Build history of the part. All positions in model axes, mm. Round coordinates to 2 decimals unless told otherwise and drop trailing zeros. Loops run counter-clockwise (first coordinate to the right, second up) from the corner with the lowest first, then second, coordinate; pieces in that order, holes last. Notation, with made-up numbers: (-10.75, 85.25) - (21.25, 85.25) arc R10 cw to (21.25, 97.25) - close; hole circle Ø7 at (5.5, 41.5). An arc over 180 degrees is marked (long way). Put each result on its own line as item: value. Start each with the question number.
Autodesk Fusion 360 part; units mm, degrees
sketch "Esquisse3" plane through (0, 0, 0) normal (0, 1, 0) x (1, 0, 0)
  line L0 (-32.5, 271.1708) -> (-7.5, 296.1708)
  line L1 (-32.5, 261.1708) -> (127.5, 261.1708) construction
  line L2 (127.5, 216.1708) -> (-32.5, 216.1708) construction
  circle A0 centre (20, 261.1708) radius 3
  line L3 (-7.5, 296.1708) -> (102.5, 296.1708)
  circle A1 centre (89.5, 194.6708) radius 3
  line L4 (-32.5, 236.1708) -> (127.5, 236.1708) construction
  line L5 (0, -4.6657) -> (95, -4.6657)
  circle A2 centre (89.5, 236.1708) radius 3
  line L6 (47.5, 23.552) -> (47.5, 296.1708)
  circle A3 centre (5.5, 194.6708) radius 3
  line L7 (47.5, 30.3343) -> (47.5, -4.6657) construction
  line L8 (-44.913, 194.6708) -> (139.913, 194.6708) construction
  line L9 (-80, 133.8984) -> (0, -4.6657)
  line L10 (95, -4.6657) -> (175, 133.8984)
  line L11 (23.75, 67.2637) -> (23.75, -4.6657) construction
  line L12 (71.25, 67.8004) -> (71.25, 0) construction
  line L13 (-32.5, 216.1708) -> (-80, 133.8984)
  line L14 (127.5, 271.1708) -> (127.5, 216.1708)
  line L15 (102.5, 296.1708) -> (127.5, 271.1708)
  line L16 (-32.5, 216.1708) -> (-32.5, 271.1708)
  line L17 (-32.5, 271.1708) -> (127.5, 271.1708) construction
  line L18 (-20.2073, 30.3343) -> (115.2073, 30.3343) construction
  line L19 (175, 133.8984) -> (127.5, 216.1708)
  circle A4 centre (75, 261.1708) radius 3
  circle A5 centre (5.5, 236.1708) radius 3
  circle A6 centre (23.75, 30.3343) radius 3
  circle A7 centre (71.25, 30.3343) radius 3
  line L20 (5.5, 300.8365) -> (5.5, 171.5052) construction
  line L21 (89.5, 296.1708) -> (89.5, 171.5052) construction
  line L22 (20, 296.1708) -> (20, 171.5052) construction
  line L23 (75, 296.1708) -> (75, 171.5052) construction
  point P0 (0, -4.6657)
  dimension "d12" = 95
  dimension "d60" = 120
  dimension "d18" = 120
  dimension "d63" = 160
  dimension "d65" = 25
  dimension "d66" = 25
  dimension "d35" = 35
  dimension "d70" = 6
  dimension "d71" = 6
  dimension "d72" = 6
  dimension "d56" = 6
  dimension "d74" = 6
  dimension "d75" = 6
  dimension "d79" = 101.5
  dimension "d80" = 23.75
  dimension "d67" = 23.75
  dimension "d88" = 80
  dimension "d89" = 60
  dimension "d90" = 25
  dimension "d95" = 95
  dimension "d96" = 160
  dimension "d97" = 35
  dimension "d98" = 6
  dimension "d99" = 6
  dimension "d100" = 38
  dimension "d101" = 38
  dimension "d102" = 52.5
  dimension "d103" = 52.5
extrude "Extrusion5" add sketch "Esquisse3" along normal blind 10.12
equation "plaque0_l1_Ref = 160 mm"
equation "plaque0_l2_Ref = 95 mm"
equation "plaque_ep = 10.12 mm"
equation "support_prof = 80 mm"
equation "support_chanf = 25 mm"
equation "trou_diam = 6.05 mm"
equation "d104 = plaque_ep"
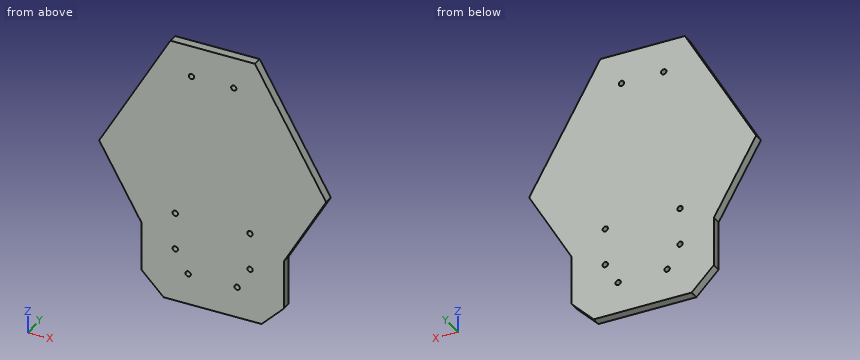
Item 1: Slice it at B-B (z = -229). Give the cut face in (x, y).
Item 2: Drill centre lines: probe 1 along Z at (x, y) = (89.5, 2.5); probe 2 along Z at (x, y) = (90.5, 7.75); probe 3 along X at (y, z) = (4, -235). Where is each one in solid material? Low to high. Write a range as [from, to].
Item 3: Drop flat-ended pins along their axis: pin 1 Ø4 at (x, z) = (69.5, -233.5) entering from -Y; pin 2 Ø4 at (y, z) = (8.5, -200) entering from +X; pin 3 Ø4 at (y, z) = (5.5, -161) entering from +X; pin 4 Ø4 at (y, z) = (1.5, -43) entering from +X. Give the stop position or say it passes through.
Item 4: Slice it at A-A (y = 6.25). Give the number of separate pieces and of enclosed holes in the cut face, plus the area to 3 significant figures.
Item 5: Slice it at C-C (x = 109.5). Give the cut face in (y, z), plus the area to 3 significant figures.
Computed values:
1. outline: (-32.5, 0) - (127.5, 0) - (127.5, 10.12) - (-32.5, 10.12) - close
2. probe 1: z = [-296.17, -239.17], [-233.17, -197.67], [-191.67, 4.67]
2. probe 2: z = [-296.17, -239], [-233.34, -197.5], [-191.84, 4.67]
2. probe 3: x = [-32.5, 2.74], [8.26, 86.74], [92.26, 127.5]
3. pin 1: stops at y = 0
3. pin 2: stops at x = 137.99
3. pin 3: stops at x = 160.51
3. pin 4: stops at x = 123.67
4. separate pieces: 1
4. enclosed holes: 8
4. area: 53,300 mm^2
5. outline: (0, -289.17) - (10.12, -289.17) - (10.12, -20.45) - (0, -20.45) - close
5. area: 2,720 mm^2
